Input: part model. Units: mm. Frame: model coordinates. A direction names the side the tool comes from. Coordinates: 2 decimals unless noted, no trailing zeros. Order: outer loops, then holes, each group sorted by start corner. A loop starts at its lowest first (then second) coordinate and runs counter-clockwise, first axis right, second up. Notation, with made-up numbers: (26.5, -21) -> (55.5, -21) arc R21 cw to (55.5, 18) -> close; hole circle Ø10 at (-19.75, 87.25). An arc over 180 degrees is marked (long way). Use CSV: the item, a comma, the result in double quotes. Start each with the question number.
```python
from build123d import *

# Parameters (mm, degrees)
SKETCH2_R           = 3.96875
BOSS_EXTRUDE1_DEPTH = 63.5
SKETCH3_R           = 3.96875


with BuildPart() as part:
    # Sketch2 → Boss-Extrude1 (new, symmetric)
    with BuildSketch(Plane.XY):
        with Locations((0, -50.8)):
            Circle(SKETCH2_R)
    extrude(amount=BOSS_EXTRUDE1_DEPTH, both=True)

    # Sweep1: sweep along a path in Sketch4
    with BuildLine(Plane(origin=(0, 0, 0), x_dir=(1, 0, 0), z_dir=(0, 1, 0))) as sweep1_path:
        Line((-19.05, -53.975), (-19.05, -63.5))
        ThreePointArc((-19.05, -63.5), (-9.525, -73.025), (0, -63.5))
    # Sketch3 → Sweep1 (sweep)
    with BuildSketch(Plane.XY.offset(63.5)):
        with Locations((0, -50.8)):
            Circle(SKETCH3_R)
    sweep(path=sweep1_path.line)


solid = part.part
```
1. Access query for faces 3 (the face through (0, -51, -63.5)), 4 (the face through (-0.517, -46.865, 0.889)). Directions: +Z, -Z, +X, -X, +Y, -Y. A direction counts if a zero-diameter tool reaches every point of the face in a straight line with its end or side. Return the directions, or none.
2. Contact query for flat-ended pins moving along their axis: P1, Ø1.5, axis at x = -11.5, y = -50, coming from the +Z side; P2, Ø6, axis at x = -9.5, z = 41.5, coming from the +Y side; P3, Ø4, axis at x = -3.5, z = 49.5, coming from the +Y side; P4, Ø1, axis at y = -49.5, z = -49, coming from the +X side. Output: stop coordinate, or through.
3. Section A-A on y = -50.8. Return loops of the section in (x, z) (1 decimal), then the cut area to 3 significant figures.
4. Section B-B on z = -45. Return loops of the section in (x, y).
5. Pull-direction query (X, two-part tool) for faces 1 (the face through (-18.19, -46.926, 58.804)), 2 (the face through (-19, -51, 53.975)); classes: released by +X, released by -X, zero draft, split by the parting line, or undercut.
6. Material intervals for line 1 along X through (y, z) = (-48.25, 65.5); line 2 along X through (y, z) = (-51.75, 62.5); line 3 along Z through (x, y) = (-4, -53), sorted ascending.
Values follow:
1,face 3,"-Z, +X, -X, +Y, -Y"
1,face 4,"-Z"
2,P1,"stops at z = 76.91"
2,P2,"passes through"
2,P3,"stops at y = -47.13"
2,P4,"stops at x = 3.89"
3,outline,"(-23, 54) -> (-15.1, 54) -> (-15.1, 63.5) arc R5.6 cw to (-4, 63.5) -> (-4, -63.5) -> (4, -63.5) -> (4, 63.5) arc R13.5 ccw to (-23, 63.5) -> close"
3,area,"1,320 mm2"
4,outline,"circle Ø7.94 at (0, -50.8)"
5,face 1,"undercut"
5,face 2,"zero draft"
6,line 1,"x = -21.93 to -15.69, -3.36 to 2.88"
6,line 2,"x = -22.9 to -15.2, -3.85 to 3.85"
6,line 3,"z = 66.36 to 75.08"
